The listing builds one solid part. Answer for the finished solid, in the listing's coordinates (mm). Give positions to 0.01 mm unless a question says otherwise; leave off trailing zeros. Loops run counter-clockwise (first coordinate to the right, second up) from the corner with the lowest first, then second, coordinate; pieces in that order, holes last. Notation, with made-up numbers: M 26,37 L 45,37 A20 cw 45,44 Z; hole C 74.5,31 d4. An arc over 180 degrees is marked long. One line per item, written item: value. Start each with the question number.
Q1. A cutting plane is placed at B-B, the plane z = 2.1. Determine the outline of the cut face in (x, y).
Q2. A cutting plane is placed at D-D, the plane y = 1.25. Determine the outline of the cut face in (x, z).
Q3. Consider L1, parallel to Y at x = -17, z = 0.9; L2, parallel to Y at x = 0, z = 2; L3, parallel to X at y = 0.75, z = 0.95. Determine where each line is inside the solid, lowest interval first.
Q4. The mould has two halves that part along Y. Classify faces 1 (the cylindrical face through (18.574, 0.496, 1.479)), 2 (the flat face through (0, -10, 1)), 3 (the cylindrical face through (-20, 0, 1)), 4 (the flat face through (0, 10, 1)): +Y half, -Y half, draft (parallel to the pull), parting line (faces both ways), or undercut.
Q5. A cutting plane is placed at A-A, the plane x = 0. Determine the outline of the cut face in (y, z).
Q6. A cutting plane is placed at C-C, the plane y = -5.25. Determine the outline of the cut face in (x, z).
from build123d import *

# Parameters (mm, degrees)
SKETCH_1_R      = 1.65
SKETCH_1_R_2    = 8.25
EXTRUDE_1_DEPTH = 3


with BuildPart() as part:
    # 草图1 → 凸台-拉伸1 (new body)
    with BuildSketch(Plane.XY):
        with BuildLine():
            ThreePointArc((-17.320508076, 10), (-20, 0), (-17.320508076, -10))
            Line((-17.320508076, -10), (17.320508076, -10))
            ThreePointArc((17.320508076, -10), (19.318516526, -5.176380902), (20, 0))
            ThreePointArc((20, 0), (19.318516526, 5.176380902), (17.320508076, 10))
            Line((17.320508076, 10), (-17.320508076, 10))
        make_face()
        with Locations((-17, 0)):
            Circle(SKETCH_1_R, mode=Mode.SUBTRACT)
        Circle(SKETCH_1_R_2, mode=Mode.SUBTRACT)
        with Locations((17, 0)):
            Circle(SKETCH_1_R, mode=Mode.SUBTRACT)
    extrude(amount=EXTRUDE_1_DEPTH)


solid = part.part
Answer block:
1. outline: M -17.32,-10 L 17.32,-10 A20 ccw 17.32,10 L -17.32,10 A20 ccw Z; hole C -17,0 d3.3; hole C 0,0 d16.5; hole C 17,0 d3.3
2. outline: M -19.96,0 L -18.08,0 L -18.08,3 L -19.96,3 Z; M -15.92,0 L -8.15,0 L -8.15,3 L -15.92,3 Z; M 8.15,0 L 15.92,0 L 15.92,3 L 8.15,3 Z; M 18.08,0 L 19.96,0 L 19.96,3 L 18.08,3 Z
3. L1: -10 to -1.65, 1.65 to 10
3. L2: -10 to -8.25, 8.25 to 10
3. L3: -19.99 to -18.47, -15.53 to -8.22, 8.22 to 15.53, 18.47 to 19.99
4. face 1: undercut
4. face 2: -Y half
4. face 3: parting line
4. face 4: +Y half
5. outline: M -10,0 L -8.25,0 L -8.25,3 L -10,3 Z; M 8.25,0 L 10,0 L 10,3 L 8.25,3 Z
6. outline: M -19.3,0 L -6.36,0 L -6.36,3 L -19.3,3 Z; M 6.36,0 L 19.3,0 L 19.3,3 L 6.36,3 Z
